```python
from build123d import *

# Parameters (mm, degrees)
F0_R     = 37
F0_R_2   = 34
F1_DEPTH = 100
F2_R     = 35.5
F3_DEPTH = 10
F4_R     = 34
F5_DEPTH = 25


with BuildPart() as f1:
    # F0 (on Front) → F1 (new body)
    with BuildSketch(Plane.XZ):
        Circle(F0_R)
        Circle(F0_R_2, mode=Mode.SUBTRACT)
    extrude(amount=-F1_DEPTH)

    # F2 (on Front) → F3 (join)
    with BuildSketch(Plane.XZ):
        Circle(F2_R)
    extrude(amount=F3_DEPTH)

    # F4 (on face) → F5 (cut)
    with BuildSketch(Plane.XZ.offset(10)):
        Circle(F4_R)
    extrude(amount=-F5_DEPTH, mode=Mode.SUBTRACT)


solid = f1.part
```
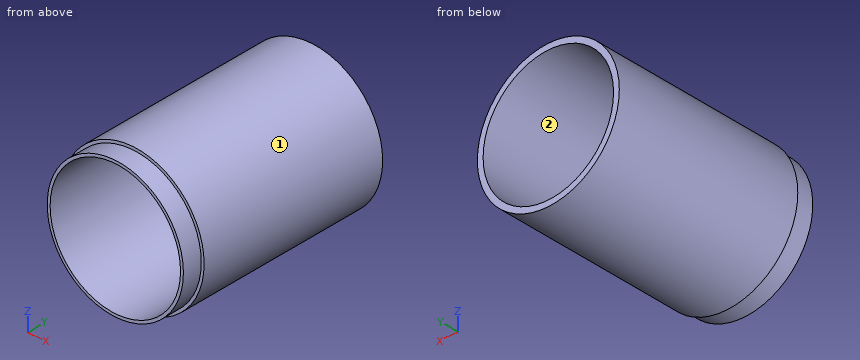
Work out the finished part from the listing and answer in its coordinate system (mm). Face numbers are marked on the shaded views. Round coordinates to 2 decimals unless told otherwise and drop trailing zeros. Order: outer loops, then holes, each group sorted by start corner. A loop starts at its lowest first (then second) coordinate and runs counter-clockwise, first axis right, second up.
Q1. Find the intervals of material crossed by line 1 along Z through (x, y) = (0, 21); line 2 along X through (y, z) = (53.5, 29.5); line 3 along Z through (x, y) = (13, 3.5), in increasing order.
Solution:
line 1: z = -37 to -34, 34 to 37
line 2: x = -22.33 to -16.9, 16.9 to 22.33
line 3: z = -34.64 to -31.42, 31.42 to 34.64
Q2. A cutting plane is placed at B-B, the plane z = 0. Determine the outline of the cut face in (x, y).
Solution:
outline: (-37, 0) - (-35.5, 0) - (-35.5, -10) - (-34, -10) - (-34, 100) - (-37, 100) - close; (34, -10) - (35.5, -10) - (35.5, 0) - (37, 0) - (37, 100) - (34, 100) - close
Q3. A cutting plane is placed at C-C, the plane y = 3.5. Determine the outline of the cut face in (x, z).
Solution:
outline: circle Ø74 at (0, 0); hole circle Ø68 at (0, 0)
Q4. The mould has two halves that part along X. Classify the marked faces 1 and 2: pulls with the +X half, pulls with the -X half, needs draft (parallel to the pull), parting line crosses it, or undercut.
Solution:
face 1: parting line crosses it
face 2: undercut
Q5. A cutting plane is placed at A-A, the plane x = 0. Determine the outline of the cut face in (y, z).
Solution:
outline: (-10, -35.5) - (0, -35.5) - (0, -37) - (100, -37) - (100, -34) - (-10, -34) - close; (-10, 34) - (100, 34) - (100, 37) - (0, 37) - (0, 35.5) - (-10, 35.5) - close
Q6. Given pin 1 Ø6 at (x, y) = (18.5, 46) entering from -Z; pin 2 Ø3 at (x, z) = (-27, -29.5) entering from -Y; pin 3 Ø5 at (x, y) = (10.5, 71) entering from -Z; pin 4 Ø6 at (x, y) = (-11.5, 76.5) entering from -Z, each flat-ended and moving along its own axis, determine where each tip first touches the part or whether it passes through.
Solution:
pin 1: stops at z = -33.6
pin 2: passes through
pin 3: stops at z = -36.12
pin 4: stops at z = -36.01
